Build history of the part. All positions in model axes, mm. A direction names the side the tool comes from. Coordinates: 2 decimals unless noted, no trailing zeros. Write each loop counter-clockwise with the first axis right and the second up, starting at its lowest first coordinate (ties: lowest second). Pieces come first, ordered by that corner, then holes.
from build123d import *

# Parameters (mm, degrees)
EXTRUDE_1_DEPTH     = 1.62
CUT_EXTRUDE_1_REACH = 3.62
SKETCH_2_R          = 1.375
SKETCH_11_W         = 51.4
SKETCH_11_H         = 5.1
EXTRUDE_9_DEPTH     = 8.45
SKETCH_12_W         = 51.4
SKETCH_12_H         = 5.1
EXTRUDE_10_DEPTH    = 10
SKETCH_13_W         = 10
SKETCH_13_H         = 13.5
SKETCH_13_W_2       = 13.5
SKETCH_13_H_2       = 10
EXTRUDE_12_DEPTH    = 6.25
SKETCH_14_W         = 13.5
SKETCH_14_H         = 0.5
CUT_EXTRUDE_2_DEPTH = 1
SKETCH_15_W         = 13.5
SKETCH_15_H         = 0.5
CUT_EXTRUDE_3_DEPTH = 1
SKETCH_16_W         = 13.5
SKETCH_16_H         = 0.5
CUT_EXTRUDE_4_DEPTH = 1
SKETCH_17_W         = 7.75
SKETCH_17_H         = 6.44
EXTRUDE_13_DEPTH    = 2.62
EXTRUDE_14_DEPTH    = 0.5
SKETCH_19_W         = 8.5
SKETCH_19_H         = 4
EXTRUDE_15_DEPTH    = 0.5
SKETCH_20_W         = 7.5
SKETCH_20_H         = 5.146384945
EXTRUDE_16_DEPTH    = 2.62
EXTRUDE_17_DEPTH    = 0.5


with BuildPart() as part:
    # 草图1 → 凸台-拉伸1 (new body)
    with BuildSketch(Plane(origin=(0, 0, 0), x_dir=(1, 0, 0), z_dir=(0, 1, 0))):
        with BuildLine():
            Line((-29.5, 15), (29.5, 15))
            ThreePointArc((29.5, 15), (31.621320344, 14.121320344), (32.5, 12))
            Line((32.5, 12), (32.5, -12))
            ThreePointArc((32.5, -12), (31.621320344, -14.121320344), (29.5, -15))
            Line((29.5, -15), (-29.5, -15))
            ThreePointArc((-29.5, -15), (-31.621320344, -14.121320344), (-32.5, -12))
            Line((-32.5, -12), (-32.5, 12))
            ThreePointArc((-32.5, 12), (-31.621320344, 14.121320344), (-29.5, 15))
        make_face()
    extrude(amount=EXTRUDE_1_DEPTH)

    # 草图2 → 切除-拉伸1 (cut, up to next)
    with BuildSketch(Plane(origin=(0, 1.62, 0), x_dir=(1, 0, 0), z_dir=(0, 1, 0)), mode=Mode.PRIVATE) as cut_extrude_1_sk1:
        with Locations(Location((29, -11.5, 0), (0, 0, 270))):  # turned: the seam where the file's is
            Circle(SKETCH_2_R)
    cut_extrude_1_tool1 = extrude(cut_extrude_1_sk1.sketch, amount=-CUT_EXTRUDE_1_REACH, mode=Mode.PRIVATE) & part.part
    add(cut_extrude_1_tool1.solids().sort_by_distance((29, 1.62, 11.5))[0], mode=Mode.SUBTRACT)
    # 草图2 → 切除-拉伸1 (cut, up to next)
    with BuildSketch(Plane(origin=(0, 1.62, 0), x_dir=(1, 0, 0), z_dir=(0, 1, 0)), mode=Mode.PRIVATE) as cut_extrude_1_sk2:
        with Locations(Location((29, 11.5, 0), (0, 0, 270))):  # turned: the seam where the file's is
            Circle(SKETCH_2_R)
    cut_extrude_1_tool2 = extrude(cut_extrude_1_sk2.sketch, amount=-CUT_EXTRUDE_1_REACH, mode=Mode.PRIVATE) & part.part
    add(cut_extrude_1_tool2.solids().sort_by_distance((29, 1.62, -11.5))[0], mode=Mode.SUBTRACT)
    # 草图2 → 切除-拉伸1 (cut, up to next)
    with BuildSketch(Plane(origin=(0, 1.62, 0), x_dir=(1, 0, 0), z_dir=(0, 1, 0)), mode=Mode.PRIVATE) as cut_extrude_1_sk3:
        with Locations(Location((-29, -11.5, 0), (0, 0, 270))):  # turned: the seam where the file's is
            Circle(SKETCH_2_R)
    cut_extrude_1_tool3 = extrude(cut_extrude_1_sk3.sketch, amount=-CUT_EXTRUDE_1_REACH, mode=Mode.PRIVATE) & part.part
    add(cut_extrude_1_tool3.solids().sort_by_distance((-29, 1.62, 11.5))[0], mode=Mode.SUBTRACT)
    # 草图2 → 切除-拉伸1 (cut, up to next)
    with BuildSketch(Plane(origin=(0, 1.62, 0), x_dir=(1, 0, 0), z_dir=(0, 1, 0)), mode=Mode.PRIVATE) as cut_extrude_1_sk4:
        with Locations(Location((-29, 11.5, 0), (0, 0, 270))):  # turned: the seam where the file's is
            Circle(SKETCH_2_R)
    cut_extrude_1_tool4 = extrude(cut_extrude_1_sk4.sketch, amount=-CUT_EXTRUDE_1_REACH, mode=Mode.PRIVATE) & part.part
    add(cut_extrude_1_tool4.solids().sort_by_distance((-29, 1.62, -11.5))[0], mode=Mode.SUBTRACT)

    # 草图11 → 凸台-拉伸9 (add)
    with BuildSketch(Plane.XZ):
        with Locations((-0.05, -11.55)):
            Rectangle(SKETCH_11_W, SKETCH_11_H)
    extrude(amount=EXTRUDE_9_DEPTH)

    # 草图12 → 凸台-拉伸10 (add)
    with BuildSketch(Plane(origin=(0, 1.62, 0), x_dir=(1, 0, 0), z_dir=(0, 1, 0))):
        with Locations((-0.05, 11.55)):
            Rectangle(SKETCH_12_W, SKETCH_12_H)
    extrude(amount=EXTRUDE_10_DEPTH)

    # 草图13 → 凸台-拉伸12 (add)
    with BuildSketch(Plane(origin=(0, 1.62, 0), x_dir=(1, 0, 0), z_dir=(0, 1, 0))):
        with Locations((-27.5, 0.12)):
            Rectangle(SKETCH_13_W, SKETCH_13_H)
        with Locations((27.5, 0.12)):
            Rectangle(SKETCH_13_W, SKETCH_13_H)
        with Locations((-8.75, -10)):
            Rectangle(SKETCH_13_W_2, SKETCH_13_H_2)
        with Locations((9.05, -10)):
            Rectangle(SKETCH_13_W_2, SKETCH_13_H_2)
    extrude(amount=EXTRUDE_12_DEPTH)

    # 草图14 → 切除-拉伸2 (cut)
    with BuildSketch(Plane.XY.offset(15)):
        with Locations((-8.75, 1.87)):
            Rectangle(SKETCH_14_W, SKETCH_14_H)
        with Locations((9.05, 1.87)):
            Rectangle(SKETCH_14_W, SKETCH_14_H)
    extrude(amount=-CUT_EXTRUDE_2_DEPTH, mode=Mode.SUBTRACT)

    # 草图15 → 切除-拉伸3 (cut)
    with BuildSketch(Plane.ZY.offset(32.5)):
        with Locations((-0.12, 1.87)):
            Rectangle(SKETCH_15_W, SKETCH_15_H)
    extrude(amount=-CUT_EXTRUDE_3_DEPTH, mode=Mode.SUBTRACT)

    # 草图16 → 切除-拉伸4 (cut)
    with BuildSketch(Plane(origin=(32.5, 0, 0), x_dir=(0, 0, -1), z_dir=(1, 0, 0))):
        with Locations((0.12, 1.87)):
            Rectangle(SKETCH_16_W, SKETCH_16_H)
    extrude(amount=-CUT_EXTRUDE_4_DEPTH, mode=Mode.SUBTRACT)

    # 草图17 → 凸台-拉伸13 (add)
    with BuildSketch(Plane(origin=(0, 1.62, 0), x_dir=(1, 0, 0), z_dir=(0, 1, 0))):
        with Locations((21.675, -11.78)):
            Rectangle(SKETCH_17_W, SKETCH_17_H)
    extrude(amount=EXTRUDE_13_DEPTH)

    # 草图18 → 凸台-拉伸14 (add)
    with BuildSketch(Plane.XY.offset(15)):
        Polygon((17.8, 2.62), (18.8, 1.62), (24.55, 1.62), (25.55, 2.62), (25.55, 3.74), (25.05, 4.24), (18.3, 4.24), (17.8, 3.74), align=None)
    extrude(amount=EXTRUDE_14_DEPTH)

    # 草图19 → 凸台-拉伸15 (add)
    with BuildSketch(Plane(origin=(0, 1.62, 0), x_dir=(1, 0, 0), z_dir=(0, 1, 0))):
        with Locations((-21.75, -11)):
            Rectangle(SKETCH_19_W, SKETCH_19_H)
    extrude(amount=EXTRUDE_15_DEPTH)

    # 草图20 → 凸台-拉伸16 (add)
    with BuildSketch(Plane.XZ):
        with Locations((9.25, 12.426807528)):
            Rectangle(SKETCH_20_W, SKETCH_20_H)
    extrude(amount=EXTRUDE_16_DEPTH)

    # 草图21 → 凸台-拉伸17 (add)
    with BuildSketch(Plane.XY.offset(15)):
        Polygon((6.5, 0), (12, 0), (13, -1), (13, -2.12), (12.5, -2.62), (6, -2.62), (5.5, -2.12), (5.5, -1), align=None)
    extrude(amount=EXTRUDE_17_DEPTH)


solid = part.part
(1) Slice it at D-D, the plane y = -4.5. List the corners of the cut face in (x, z), and give its area (3 significant figures).
(2) Flat gauge pins, fed straight in: P1, Ø3, axis at x = 6, y = 5, coming from the +Z side; P2, Ø4.5, axis at x = -22, z = 10, coming from the +Y side; P3, Ø1, axis at x = -3.5, z = -2.5, coming from the -Y side. Where does each tip first touch, or does it go through?
(3) Slice it at C-C, the plane z = -11. List the corners of the cut face in (x, y), and give its area (3 significant figures).
(4) 3-axis set-ups, long thin cutter, end or side, ignore diameter. For faces 4 (the flat face through (-15.5, 5, 10)), 5 (the flat face through (22, 4.24, 12)), 6 (the flat face through (-28, 5, -6.87)), 7 (the flat face through (-9, 5, 5)), 8 (the flat face through (-9, 7.87, 10)): which of +Z, -Z, +X, -X, +Y, -Y reach the whole face in a straight line?
(5) Two-plate mould, pull along Z, no slides. Class faces 1 (the flat face through (27, 5, 6.63)), 2 (the flat face through (9, 7.87, 10)), 3 (the flat face through (-9, 5, 15)): pulls with the +Z half, pulls with the -Z half, needs draft (parallel to the pull), parting line crosses it, or undercut.
(6) Slice it at B-B, the plane x = -5. List the corners of the cut face in (y, z).
(7) Slice it at A-A, the plane z = 0. List the corners of the cut face in (x, y).
(8) Probe L1, parallel to X at y = 0.75, z = 11.5 (3 decimals); L2, parallel to X at y = 7.5, z = 14; L3, parallel to X at y = 3, z = -5.5. List the from-to ranges inside material, lowest first.
Results:
1. outline: (-25.75, -14.1) - (25.65, -14.1) - (25.65, -9) - (-25.75, -9) - close
1. area: 262 mm2
2. P1: stops at z = 15
2. P2: stops at y = 2.12
2. P3: stops at y = 0
3. outline: (-32.5, 0) - (-30.28, 0) - (-30.28, 1.62) - (-32.5, 1.62) - close; (-27.72, 0) - (-25.75, 0) - (-25.75, -8.45) - (25.65, -8.45) - (25.65, 0) - (27.72, 0) - (27.72, 1.62) - (25.65, 1.62) - (25.65, 11.62) - (-25.75, 11.62) - (-25.75, 1.62) - (-27.72, 1.62) - close; (30.28, 0) - (32.5, 0) - (32.5, 1.62) - (30.28, 1.62) - close
3. area: 1,050 mm2
4. face 4: +Z, +Y
4. face 5: +Z, +X, +Y
4. face 6: +X, -X, +Y
4. face 7: +Y
4. face 8: +Z, +X, -X, +Y
5. face 1: undercut
5. face 2: needs draft
5. face 3: pulls with the +Z half
6. outline: (-8.45, -14.1) - (0, -14.1) - (0, -15) - (1.62, -15) - (1.62, -14.1) - (11.62, -14.1) - (11.62, -9) - (1.62, -9) - (1.62, 5) - (7.87, 5) - (7.87, 15) - (2.12, 15) - (2.12, 14) - (1.62, 14) - (1.62, 15) - (0, 15) - (0, -9) - (-8.45, -9) - close
7. outline: (-32.5, 0) - (32.5, 0) - (32.5, 1.62) - (31.5, 1.62) - (31.5, 2.12) - (32.5, 2.12) - (32.5, 7.87) - (22.5, 7.87) - (22.5, 1.62) - (-22.5, 1.62) - (-22.5, 7.87) - (-32.5, 7.87) - (-32.5, 2.12) - (-31.5, 2.12) - (-31.5, 1.62) - (-32.5, 1.62) - close
8. L1: x = -32.5 to -30.375, -27.625 to 27.625, 30.375 to 32.5
8. L2: x = -15.5 to -2, 2.3 to 15.8
8. L3: x = -32.5 to -22.5, 22.5 to 32.5
